```python
from build123d import *

# Parameters (mm, degrees)
SKETCH1_R                 = 4.35
BOSS_EXTRUDE1_DEPTH       = 10
CUT_EXTRUDE1_DEPTH        = 135
SKETCH3_W                 = 83.5
SKETCH3_H                 = 2.3
CUT_EXTRUDE2_DEPTH        = 135
LPATTERN1_COUNT           = 3
LPATTERN1_PITCH           = 4.3
CUT_EXTRUDE3_DEPTH        = 1
SKETCH5_W                 = 25
SKETCH5_H                 = 15
BOSS_EXTRUDE2_DEPTH       = 20
F_6_CLEARANCE_HOLE1_D     = 4.3053
F_6_CLEARANCE_HOLE1_DEPTH = 20
F_6_CLEARANCE_HOLE1_TIP   = 1.293442612


with BuildPart() as part:
    # Sketch1 → Boss-Extrude1 (new, symmetric)
    with BuildSketch(Plane.XY):
        with BuildLine():
            Line((-77.5, 0), (77.5, 0))
            Line((77.5, 0), (77.5, 7.5))
            ThreePointArc((77.5, 7.5), (75.303300859, 12.803300859), (70, 15))
            Line((70, 15), (50, 15))
            Line((50, 15), (50, 145))
            Line((50, 145), (-50, 145))
            Line((-50, 145), (-50, 15))
            Line((-50, 15), (-70, 15))
            ThreePointArc((-70, 15), (-75.303300859, 12.803300859), (-77.5, 7.5))
            Line((-77.5, 7.5), (-77.5, 0))
        make_face()
        with Locations((-70, 7.5)):
            Circle(SKETCH1_R, mode=Mode.SUBTRACT)
        with Locations((70, 7.5)):
            Circle(SKETCH1_R, mode=Mode.SUBTRACT)
    extrude(amount=BOSS_EXTRUDE1_DEPTH, both=True)

    # Sketch2 → Cut-Extrude1 (cut)
    with BuildSketch(Plane(origin=(0, 145, 0), x_dir=(1, 0, 0), z_dir=(0, 1, 0))):
        Polygon((-40.625, -10), (-40.625, 6.28), (-42.625, 6.28), (-42.625, 8.08), (-40.625, 8.08), (-40.625, 10), (40.625, 10), (40.625, 8.08), (42.625, 8.08), (42.625, 6.28), (40.625, 6.28), (40.625, -10), align=None)
    extrude(amount=-CUT_EXTRUDE1_DEPTH, mode=Mode.SUBTRACT)

    # Sketch3 → Cut-Extrude2 (cut)
    with BuildSketch(Plane(origin=(0, 145, 0), x_dir=(1, 0, 0), z_dir=(0, 1, 0))):
        with Locations((0, 2.63)):
            Rectangle(SKETCH3_W, SKETCH3_H)
    cut_extrude2 = extrude(amount=-CUT_EXTRUDE2_DEPTH, mode=Mode.SUBTRACT)

    # LPattern1: Cut-Extrude2 ×3
    with Locations(*[(0, 0, i * LPATTERN1_PITCH) for i in range(1, LPATTERN1_COUNT)]):
        add(cut_extrude2, mode=Mode.SUBTRACT)

    # Sketch4 → Cut-Extrude3 (cut)
    with BuildSketch(Plane(origin=(0, 15, 0), x_dir=(1, 0, 0), z_dir=(0, 1, 0))):
        Polygon((60, 7.5), (55.5, 0.5), (58.5, 0.5), (58.5, -7.5), (61.5, -7.5), (61.5, 0.5), (64.5, 0.5), align=None)
    cut_extrude3 = extrude(amount=-CUT_EXTRUDE3_DEPTH, mode=Mode.SUBTRACT)

    # Mirror1: Cut-Extrude3 across plane
    add(cut_extrude3.mirror(Plane(origin=(0, 0, 0), x_dir=(0, 0, 1), z_dir=(1, 0, 0))), mode=Mode.SUBTRACT)

    # Sketch5 → Boss-Extrude2 (add)
    with BuildSketch(Plane(origin=(0, 0, -10), x_dir=(-1, 0, 0), z_dir=(0, 0, -1))):
        with Locations((-62.5, 112.5)):
            Rectangle(SKETCH5_W, SKETCH5_H)
    extrude(amount=-BOSS_EXTRUDE2_DEPTH)

    # #6 Clearance Hole1
    with Locations(Plane(origin=(0, 120, 0), x_dir=(1, 0, 0), z_dir=(0, 1, 0))):
        with Locations((70, 5), (70, -5)):
            Hole(F_6_CLEARANCE_HOLE1_D / 2, depth=F_6_CLEARANCE_HOLE1_DEPTH)
            with Locations((0, 0, -(F_6_CLEARANCE_HOLE1_DEPTH + F_6_CLEARANCE_HOLE1_TIP / 2))):  # 118° drill point
                Cone(0, F_6_CLEARANCE_HOLE1_D / 2, F_6_CLEARANCE_HOLE1_TIP, mode=Mode.SUBTRACT)


solid = part.part
```
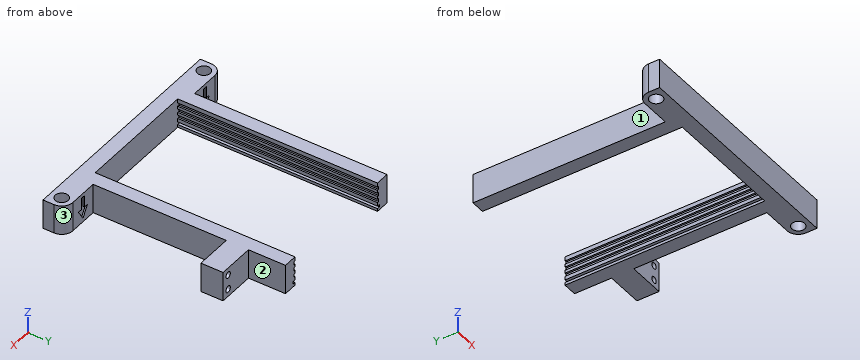
Verification items for the finished model (mm, model axes). Face numbers are marked on the shaded views. A direction names the side the tool comes from. Round coordinates to 2 decimals unless told otherwise and drop trailing zeros. Write each loop counter-clockwise with the first axis right and the second up, starting at its lowest first coordinate (ties: lowest second). Pieces come first, ordered by that corner, then holes. Notation, with made-up numbers: (-40, 46) - (1, 46) arc R17 ccw to (1, 73) - close; hole circle Ø3 at (87, 51). An arc over 180 degrees is marked (long way). Answer as a JSON object with one key per item and string values. Group by question number.
Q1. Section check B-B, the plane x = -53. Enter the section's corners in (y, z), plus the area to 3 significant figures.
Q2. Tool access check on the marked faces 1, 2 and 3. Record the directions out of +Z, -Z, +X, -X, +Y, -Y that give a thin tool (end or side, any length) a straight path to the whole face; none if there is none.
Q3. Go/stop test with flat-tipped pins: pin 1 Ø5 at (y, z) = (16, 0) entering from -X; pin 2 Ø0.7 at (y, z) = (67.5, -2.5) entering from -X; pin 3 Ø0.8 at (y, z) = (14.5, 2) entering from -X. Record where each tip stops, or that it passes through.
Q4. Thickness scan on line 1 (Z direction, x = 70, y = 109); line 2 (X direction, y = 61.5, z = 7.75) (3 decimals); line 3 (X direction, y = 47, z = 6.25). Record the ranges inside material, lowest first.
Q5. Section check A-A, the plane x = -22.5. Enter the section's corners in (y, z).
Found:
{
 "1": {"outline": "(0, -10) - (15, -10) - (15, 10) - (0, 10) - close", "area": "300 mm^2"},
 "2": {"face 1": "+Z, -Z, -X, +Y", "face 2": "+Z, -Z, +X, +Y", "face 3": "+Z, -Z, +X"},
 "3": {"pin 1": "stops at x = -74.5", "pin 2": "stops at x = -50", "pin 3": "stops at x = -73.56"},
 "4": {"line 1": "z = -10 to -7.15, -2.85 to 2.85, 7.15 to 10", "line 2": "x = -50 to -40.625, 40.625 to 50", "line 3": "x = -50 to -41.75, 41.75 to 50"},
 "5": {"outline": "(0, -10) - (10, -10) - (10, 10) - (0, 10) - close"}
}
